Source: CAD feature listing. Evaluate the final solid. Frame: model axes, mm. Coordinates: 2 decimals unless noted, no trailing zeros. Order: outer loops, then holes, each group sorted by start corner. A loop starts at its lowest first (then second) coordinate and runs counter-clockwise, first axis right, second up. Notation, with made-up numbers: (-13.5, -14) -> (17.5, -14) arc R17 cw to (17.5, 18) -> close; hole circle Ø11 at (-18, -9.5). An arc over 180 degrees is marked (long way). Put each result on its own line as item: value.
from build123d import *

# Parameters (mm, degrees)
F0_W     = 7
F0_H     = 30
F1_DEPTH = 2
F2_R     = 1.5
F3_DEPTH = 40
F4_R     = 1


with BuildPart() as f1:
    # F0 (on Front) → F1 (new body)
    with BuildSketch(Plane.XZ):
        Rectangle(F0_W, F0_H)
    extrude(amount=F1_DEPTH)

    # F2 (on face) → F3 (join)
    with BuildSketch(Plane.XZ.offset(2)):
        Circle(F2_R)
    extrude(amount=F3_DEPTH)

    # F4
    f4_edges = [f1.edges().sort_by_distance(p)[0] for p in [
        (-1.5, -42, 0),
    ]]
    fillet(f4_edges, radius=F4_R)


solid = f1.part
1. Cut plane B-B on y = -22. Output: boundary loops of the cut face in (x, z), plus the area to 3 significant figures.
Numbers:
outline: circle Ø3 at (0, 0)
area: 7.07 mm2
2. Cut plane C-C on z = -2.75. Output: boundary loops of the cut face in (x, y), plus the area to 3 significant figures.
Numbers:
outline: (-3.5, -2) -> (3.5, -2) -> (3.5, 0) -> (-3.5, 0) -> close
area: 14.0 mm2
3. First-contact query: pin 1 (4 mm diameter, centred on y = -33.5, z = 1, fed in from -X); pin 2 (3 mm diameter, centred on y = -26, z = -0.5, fed in from +X). Flat tips, straight axial feed; report the tip coordinate or a pass-through.
Numbers:
pin 1: stops at x = -1.5
pin 2: stops at x = 1.5
4. Ray query, line 1 along Y through (x, z) = (-1.5, -10.25); line 2 along Z through (x, y) = (1.25, -15.5); line 3 along Z through (x, y) = (-0.25, -40). Return the intervals inside material, ascending.
Numbers:
line 1: y = -2 to 0
line 2: z = -0.83 to 0.83
line 3: z = -1.48 to 1.48
5. Pull-direction query (X, two-part tool) for faces 1 (the cylindrical face through (-1.5, -21.23, 0.07)), 2 (the flat face through (-2, -2, 0)), 3 (the flat face through (3.5, -1, 0)); classes: pulls with the +X half, pulls with the -X half, needs draft (parallel to the pull), parting line crosses it, or undercut.
Numbers:
face 1: parting line crosses it
face 2: needs draft
face 3: pulls with the +X half
6. Cut plane A-A on x = 3. Output: boundary loops of the cut face in (y, z), plus the area to 3 significant figures.
Numbers:
outline: (-2, -15) -> (0, -15) -> (0, 15) -> (-2, 15) -> close
area: 60.0 mm2
